from build123d import *

# Parameters (mm, degrees)
F1_DEPTH = 50.8
F2_R     = 2.4892
F3_DEPTH = 25.4
F4_R     = 3.175
F5_DEPTH = 25.4


with BuildPart() as f1:
    # F0 (on Top) → F1 (new body)
    with BuildSketch(Plane.XY):
        Polygon((3.175, 25.4), (0, 25.4), (0, 0), (25.4, 0), (25.4, 3.175), (3.175, 3.175), align=None)
    extrude(amount=F1_DEPTH)

    # F2 (on face) → F3 (cut)
    with BuildSketch(Plane.XZ):
        with Locations((12.7, 38.1)):
            Circle(F2_R)
        with Locations((12.7, 12.7)):
            Circle(F2_R)
    extrude(amount=-F3_DEPTH, mode=Mode.SUBTRACT)

    # F4 (on face) → F5 (cut)
    with BuildSketch(Plane(origin=(0, 0, 0), x_dir=(0, -1, 0), z_dir=(-1, 0, 0))):
        with Locations((-6.35, 25.4)):
            Circle(F4_R)
    extrude(amount=-F5_DEPTH, mode=Mode.SUBTRACT)


solid = f1.part
Input: part model. Units: mm. Frame: model coordinates. A direction names the side the tool comes from. Give positions to 0.01 mm unless a question says otherwise; leave off trailing zeros. Order: outer loops, then holes, each group sorted by start corner. A loop starts at its lowest first (then second) coordinate and runs counter-clockwise, first axis right, second up. Notation, with made-up numbers: (21.5, -34.5) -> (29.5, -34.5) arc R29 cw to (29.5, -8.5) -> close; hole circle Ø10 at (-7, 21.25). An arc over 180 degrees is marked (long way). Use one line per item in the form item = value.
1) Section D-D, the plane y = 7.25. Return loops of the section in (x, z) (3 decimals).
Response values:
outline = (0, 0) -> (3.175, 0) -> (3.175, 22.355) -> (0, 22.355) -> close; (0, 28.445) -> (3.175, 28.445) -> (3.175, 50.8) -> (0, 50.8) -> close
2) Section A-A, the plane z = 38.1. Return loops of the section in (x, y) (3 decimals).
Response values:
outline = (0, 0) -> (10.211, 0) -> (10.211, 3.175) -> (3.175, 3.175) -> (3.175, 25.4) -> (0, 25.4) -> close; (15.189, 0) -> (25.4, 0) -> (25.4, 3.175) -> (15.189, 3.175) -> close
3) Section B-B, the plane x = 12.7. Return loops of the section in (y, z) (3 decimals).
Response values:
outline = (0, 0) -> (3.175, 0) -> (3.175, 10.211) -> (0, 10.211) -> close; (0, 15.189) -> (3.175, 15.189) -> (3.175, 35.611) -> (0, 35.611) -> close; (0, 40.589) -> (3.175, 40.589) -> (3.175, 50.8) -> (0, 50.8) -> close
4) Line query: probe 1 along Z at (x, y) = (12.7, 2.55); probe 2 along X at (y, z) = (19.5, 28) (3 decimals). Output: solid intervals per line, ascending.
Response values:
probe_1 = 0 to 10.21, 15.19 to 35.61, 40.59 to 50.8
probe_2 = 0 to 3.175
5) First-contact query: pin 1 Ø10 at (x, y) = (9, 22) entering from -Z; pin 2 Ø6 at (x, z) = (22, 14) entering from +Y (3 decimals); pin 3 Ø6.5 at (y, z) = (16.5, 13) entering from +X (3 decimals). Flat tips, straight axial feed; report the tip coordinate or a pass-through.
Response values:
pin_1 = through
pin_2 = 3.175
pin_3 = 3.175
6) Reachability of faces 4 (the flat face through (14, 3.175, 25)), 5 (the flat face through (0, 13, 25)) from +Z, -Z, +X, -X, +Y, -Y: full face, straight path, thin tool, end or side. Return the list, or none.
Response values:
face_4 = +Z, -Z, +X, +Y
face_5 = +Z, -Z, -X, +Y, -Y
7) Mould query, pull axis Z, two halves, no side actions, for faces 1 (the cylindrical face through (1.57, 6.76, 28.55)), 2 (the flat face through (7, 2, 0)), 3 (the flat face through (3.175, 14, 25)). Classes: pulls with the +Z half, pulls with the -Z half, needs draft (parallel to the pull), parting line crosses it, or undercut.
Response values:
face_1 = undercut
face_2 = pulls with the -Z half
face_3 = needs draft
8) Section C-C, the plane y = 2.5. Return loops of the section in (x, z), and give its area (3 significant figures).
Response values:
outline = (0, 0) -> (25.4, 0) -> (25.4, 50.8) -> (0, 50.8) -> close; hole circle Ø4.98 at (12.7, 12.7); hole circle Ø4.98 at (12.7, 38.1)
area = 1,250 mm^2
